Model file for the job. Use its own axes, mm. A direction names the side the tool comes from. Give positions to 0.01 mm unless a question says otherwise; leave off trailing zeros. Write each loop counter-clockwise with the first axis right and the second up, starting at its lowest first coordinate (ties: lowest second). Pieces come first, ordered by that corner, then holes. Notation, with made-up numbers: (73.25, 17.5) - (97.25, 17.5) arc R22 ccw to (97.25, 52.5) - close; hole circle Ø10 at (83, 62). An arc over 180 degrees is marked (long way). Use CSV: the item, a comma, the result in double quotes.
Autodesk Inventor part; units mm, degrees
ref_plane "YZ Plane" through (0, 0, 0) normal (1, 0, 0) x (0, 1, 0)
ref_plane "XZ Plane" through (0, 0, 0) normal (0, 1, 0) x (-1, 0, 0)
ref_plane "XY Plane" through (0, 0, 0) normal (0, 0, 1) x (1, 0, 0)
sketch "Boceto1" plane through (0, 0, 0) normal (0, 1, 0) x (-1, 0, 0)
  line L0 (-420, 120) -> (-420, -140)
  circle A0 centre (-50, -70) radius 3
  circle A1 centre (-10, -70) radius 5
  line L1 (-200, -140) -> (-200, 120)
  circle A2 centre (-50, -70) radius 50
  line L2 (-200, -20) -> (-50, -20)
  line L3 (-200, -120) -> (-50, -120)
  line L4 (-200, -140) -> (-420, -140)
  line L5 (-420, 120) -> (-200, 120)
  circle A3 centre (-50, -70) radius 3.5
  arc A4 (-52.881, -68.0126) -> (-46.5233, -70.4029) centre (-50, -70) ccw
  line L6 (-50, -70) -> (-52.881, -68.0126) construction
  line L7 (-50, -70) -> (-46.5233, -70.4029) construction
  arc A5 (-48.0126, -67.119) -> (-49.5971, -66.5233) centre (-50, -70) ccw
  line L8 (-50, -70) -> (-49.5971, -66.5233) construction
  line L9 (-50, -70) -> (-48.0126, -67.119) construction
  line L10 (-46.5233, -70.4029) -> (-48.0126, -67.119)
  line L11 (-49.5971, -66.5233) -> (-52.881, -68.0126)
  point P0 (0, 0)
  dimension "d1" = 260
  dimension "d10" = 6
  dimension "d14" = 10
  dimension "d22" = 40
  dimension "d29" = 220
  dimension "d43" = 100
  dimension "d51" = 20
  dimension "d52" = 200
  dimension "d58" = 7
  dimension "d63" = 207.99
  dimension "d64" = 27.99
  dimension "d71" = 20
extrude "Extrusión2" add sketch "Boceto1" along normal blind 10 contours L5 L1 L4 L0 | L2 A2 L3 L1 | A2 | A0 | A0 L10 A3 L11 | L10 A3 | A0 L11 A3 L10 | L11 A3 | A1
extrude "Extrusión4" cut sketch "Boceto1" along normal blind 10 contours A1
extrude "Extrusión5" cut sketch "Boceto1" along normal blind 10 contours A0 | A0 L10 A3 L11 | A0 L11 A3 L10
properties part number "Posicionador" material "Acero, fundido"
(1) Wall check: probe 1 along X at (y, z) = (3.5, 108); probe 2 along Z at (x, y) = (10, 3); probe 3 along Z at (x, y) = (50, 5.25). Give the ranges that are in metal, low to high. Write a range as [from, to].
Checked values:
probe 1,"x = [200, 420]"
probe 2,"z = [-100, -75], [-65, -40]"
probe 3,"z = [-120, -73.5], [-66.71, -20]"
(2) Flat gauge pins, fed straight in: P1, Ø5, axis at x = 141.5, y = 1.5, coming from the +Z side; P2, Ø12, axis at x = 185, z = -42.5, coming from the -Y side; P3, Ø5, axis at y = 7.5, z = -126, coming from the -X side; P4, Ø4, axis at x = 50, z = -70, coming from the +Y side. Where does each tip first touch, or does it go through?
Checked values:
P1,"stops at z = -20"
P2,"stops at y = 0"
P3,"stops at x = 200"
P4,"passes through"
(3) Saw through at A-A, the plane y = 1.75. List the corners of the cut face in (x, z).
Checked values:
outline,"(50, -120) - (200, -120) - (200, -140) - (420, -140) - (420, 120) - (200, 120) - (200, -20) - (50, -20) arc R50 ccw to start; hole circle Ø10 at (10, -70); hole (46.52, -70.4) arc R3.5 ccw (long way) to (52.88, -68.01) - (49.6, -66.52) arc R3.5 ccw to (48.01, -67.12) - close"
(4) 3-axis set-ups, long thin cutter, end or side, ignore diameter. For faces 1 (the face through (308, 5, -140)), 2 (the face through (200, 5, -130)), 3 (the face through (126, 5, -20)): which of +Z, -Z, +X, -X, +Y, -Y reach the whole face in a straight line?
Checked values:
face 1,"-Z, +X, -X, +Y, -Y"
face 2,"-Z, -X, +Y, -Y"
face 3,"+Z, -X, +Y, -Y"
(5) Pull direction Z, two halves, no side cores. Call faces 4 (the face through (260, 10, -8)), 5 (the face through (5.23, 4.93, -71.5)), 6 (the face through (0.012, 4.93, -68.901)): released by +Z, released by -Z, zero draft, split by the parting line, or undercut.
Checked values:
face 4,"zero draft"
face 5,"undercut"
face 6,"split by the parting line"
(6) Saw through at B-B, the plane z = 49.5. List the corners of the cut face in (x, y).
Checked values:
outline,"(200, 0) - (420, 0) - (420, 10) - (200, 10) - close"
